Here's how the part is built. I have some questions about the finished solid (model axes, mm). A direction names the side the tool comes from. Coordinates: 2 decimals unless noted, no trailing zeros. Loops run counter-clockwise (first coordinate to the right, second up) from the corner with the lowest first, then second, coordinate; pieces in that order, holes last.
```python
from build123d import *

# Parameters (mm, degrees)
ESQUISSE1_R           = 27
ESQUISSE1_R_2         = 15
EXTRUSION1_DEPTH      = 160
ESQUISSE2_R           = 2
EXTRUSION2_DEPTH      = 15
ESQUISSE3_R           = 2
EXTRUSION3_DEPTH      = 15
ESQUISSE4_R           = 17
ESQUISSE4_R_2         = 15
EXTRUSION4_DEPTH      = 2.5
ESQUISSE5_R           = 17
ESQUISSE5_R_2         = 15
EXTRUSION5_DEPTH      = 2.5
ESQUISSE6_W           = 120
ESQUISSE6_H           = 6
EXTRUSION6_DEPTH      = 28
EXTRUSION6_DEPTH_BACK = 28
ESQUISSE7_W           = 7
ESQUISSE7_H           = 10
EXTRUSION7_DEPTH      = 28
EXTRUSION7_DEPTH_BACK = 28


with BuildPart() as part:
    # Esquisse1 → Extrusion1 (new body)
    with BuildSketch(Plane.XY):
        Circle(ESQUISSE1_R)
        Circle(ESQUISSE1_R_2, mode=Mode.SUBTRACT)
    extrude(amount=EXTRUSION1_DEPTH)

    # Esquisse2 → Extrusion2 (cut)
    with BuildSketch(Plane.XY.offset(160)):
        with Locations((16.970013406, 16.971095673)):
            Circle(ESQUISSE2_R)
        with Locations((16.970013406, -16.970029824)):
            Circle(ESQUISSE2_R)
        with Locations((-16.971112091, -16.970029824)):
            Circle(ESQUISSE2_R)
        with Locations((-16.971112091, 16.971095673)):
            Circle(ESQUISSE2_R)
    extrude(amount=-EXTRUSION2_DEPTH, mode=Mode.SUBTRACT)

    # Esquisse3 → Extrusion3 (cut)
    with BuildSketch(Plane(origin=(0, 0, 0), x_dir=(-1, 0, 0), z_dir=(0, 0, -1))):
        with Locations((16.970013406, 16.971095673)):
            Circle(ESQUISSE3_R)
        with Locations((-16.971112091, 16.971095673)):
            Circle(ESQUISSE3_R)
        with Locations((-16.971112091, -16.970029824)):
            Circle(ESQUISSE3_R)
        with Locations((16.970013406, -16.970029824)):
            Circle(ESQUISSE3_R)
    extrude(amount=-EXTRUSION3_DEPTH, mode=Mode.SUBTRACT)

    # Esquisse4 → Extrusion4 (cut)
    with BuildSketch(Plane.XY.offset(160)):
        Circle(ESQUISSE4_R)
        Circle(ESQUISSE4_R_2, mode=Mode.SUBTRACT)
    extrude(amount=-EXTRUSION4_DEPTH, mode=Mode.SUBTRACT)

    # Esquisse5 → Extrusion5 (cut)
    with BuildSketch(Plane(origin=(0, 0, 0), x_dir=(-1, 0, 0), z_dir=(0, 0, -1))):
        Circle(ESQUISSE5_R)
        Circle(ESQUISSE5_R_2, mode=Mode.SUBTRACT)
    extrude(amount=-EXTRUSION5_DEPTH, mode=Mode.SUBTRACT)

    # Esquisse6 → Extrusion6 (cut, two sides)
    with BuildSketch(Plane(origin=(0, 0, 0), x_dir=(0, 0, -1), z_dir=(1, 0, 0))) as extrusion6_sk:
        with Locations((-80, -24)):
            Rectangle(ESQUISSE6_W, ESQUISSE6_H)
    extrude(amount=EXTRUSION6_DEPTH, mode=Mode.SUBTRACT)
    extrude(extrusion6_sk.sketch, amount=-EXTRUSION6_DEPTH_BACK, mode=Mode.SUBTRACT)

    # Esquisse7 → Extrusion7 (cut, two sides)
    with BuildSketch(Plane(origin=(0, 0, 0), x_dir=(1, 0, 0), z_dir=(0, 1, 0))) as extrusion7_sk:
        with Locations((23.5, -150)):
            Rectangle(ESQUISSE7_W, ESQUISSE7_H)
        with Locations((-23.5, -150)):
            Rectangle(ESQUISSE7_W, ESQUISSE7_H)
    extrude(amount=EXTRUSION7_DEPTH, mode=Mode.SUBTRACT)
    extrude(extrusion7_sk.sketch, amount=-EXTRUSION7_DEPTH_BACK, mode=Mode.SUBTRACT)


solid = part.part
```
1. We'd pull the mould along Y, two halves only. Please class faces 4 (the flat face through (0, -21, 81)), 5 (the flat face through (6, -14, 157.5)), 6 (the flat face through (-23, 0, 155)): +Y half, -Y half, draft (parallel to the pull), parting line (faces both ways), or undercut.
2. I want a section at D-D (z = 17). Please give me the cut outline in (x, y), then the cut area to 3 significant figures.
3. I need wall thicknesses on line 1 along Y through (x, z) = (0, 78); line 2 along Z through (x, y) = (23, -6.5); line 3 along Z through (x, y) = (-5.5, -25). Which ranges of each line are inside material? Lowest first, please.
4. For pin 1 (4 mm diameter, centred on y = 19, z = 94, fed in from -X); pin 2 (5 mm diameter, centred on y = -19, z = 80, fed in from +X); pin 3 (3.5 mm diameter, centred on x = -16.97, y = -16.97, fed in from -Z), each with a flat end and sliding along its axis, tell me the tip position at first contact or that it passes through.
5. I want a section at B-B (y = 0). Please give me the cut outline in (x, z).
6. I want a section at C-C (x = 9). Please give me the cut outline in (y, z), then the cut area to 3 significant figures.
7. I want a section at A-A (x = 0). Please give me the cut outline in (y, z).
8. On a 3-axis mill with a long thin cutter (end or side, diameter ignored), from which of +Z, -Z, +X, -X, +Y, -Y can I reach the whole of each face in a straight line? I mean faces 1 (the flat face through (20, 0, 150)), 2 (the cylindrical face through (-18.045, -15.284, 7.395)), 3 (the flat face through (17, -17, 145)). Say none if no direction works.
Response values:
1. face 4: -Y half
1. face 5: undercut
1. face 6: draft
2. outline: circle Ø54 at (0, 0); hole circle Ø30 at (0, 0)
2. area: 1,580 mm2
3. line 1: y = -21 to -15, 15 to 27
3. line 2: z = 0 to 145, 155 to 160
3. line 3: z = 0 to 20, 140 to 160
4. pin 1: stops at x = -20.98
4. pin 2: stops at x = 21.37
4. pin 3: stops at z = 15
5. outline: (-27, 0) - (-17, 0) - (-17, 2.5) - (-15, 2.5) - (-15, 157.5) - (-17, 157.5) - (-17, 160) - (-27, 160) - (-27, 155) - (-20, 155) - (-20, 145) - (-27, 145) - close; (15, 2.5) - (17, 2.5) - (17, 0) - (27, 0) - (27, 145) - (20, 145) - (20, 155) - (27, 155) - (27, 160) - (17, 160) - (17, 157.5) - (15, 157.5) - close
6. outline: (-25.46, 0) - (-14.42, 0) - (-14.42, 2.5) - (-12, 2.5) - (-12, 157.5) - (-14.42, 157.5) - (-14.42, 160) - (-25.46, 160) - (-25.46, 140) - (-21, 140) - (-21, 20) - (-25.46, 20) - close; (12, 2.5) - (14.42, 2.5) - (14.42, 0) - (25.46, 0) - (25.46, 160) - (14.42, 160) - (14.42, 157.5) - (12, 157.5) - close
6. area: 3,750 mm2
7. outline: (-27, 0) - (-17, 0) - (-17, 2.5) - (-15, 2.5) - (-15, 157.5) - (-17, 157.5) - (-17, 160) - (-27, 160) - (-27, 140) - (-21, 140) - (-21, 20) - (-27, 20) - close; (15, 2.5) - (17, 2.5) - (17, 0) - (27, 0) - (27, 160) - (17, 160) - (17, 157.5) - (15, 157.5) - close
8. face 1: +X, +Y, -Y
8. face 2: -Z
8. face 3: +Z
